```python
from build123d import *

# Parameters (mm, degrees)
SKETCH1_W                = 14.684375
SKETCH1_H                = 14.684375
BOSS_EXTRUDE1_DEPTH      = 446.0875
SKETCH9_R                = 3.384543224
CUT_EXTRUDE1_DEPTH       = 447.389511797
BOSS_EXTRUDE7_DEPTH      = 155
BOSS_EXTRUDE7_DEPTH_BACK = 155
BOSS_EXTRUDE8_DEPTH      = 164
BOSS_EXTRUDE8_DEPTH_BACK = 164
BOSS_EXTRUDE9_DEPTH      = 164
BOSS_EXTRUDE9_DEPTH_BACK = 164


with BuildPart() as part:
    # Sketch1 → Boss-Extrude1 (new body)
    with BuildSketch(Plane.XY):
        Rectangle(SKETCH1_W, SKETCH1_H)
    extrude(amount=BOSS_EXTRUDE1_DEPTH)

    # Sketch9 → Cut-Extrude1 (cut, through all)
    with BuildSketch(Plane(origin=(0, 7.3421875, 0), x_dir=(1, 0, 0), z_dir=(0, 1, 0))):
        with Locations(Location((0, -25.4, 0), (0, 0, 270))):
            Circle(SKETCH9_R)
        with Locations(Location((0, -66.675, 0), (0, 0, 270))):
            Circle(SKETCH9_R)
    extrude(amount=-CUT_EXTRUDE1_DEPTH, mode=Mode.SUBTRACT)

    # Sketch3 → Boss-Extrude7 (add, two sides: drawn at the far end of the back side and taken through both)
    with BuildSketch(Plane(origin=(0, 0, 0), x_dir=(0, 0, -1), z_dir=(1, 0, 0)).offset(-BOSS_EXTRUDE7_DEPTH_BACK)):
        with BuildLine():
            ThreePointArc((-417.5125, 0), (-422.275, 4.7625), (-427.0375, 0))
            Line((-427.0375, 0), (-417.5125, 0))
        make_face()
        with BuildLine():
            Line((-417.5125, 0), (-427.0375, 0))
            ThreePointArc((-427.0375, 0), (-422.275, -4.7625), (-417.5125, 0))
        make_face()
    extrude(amount=BOSS_EXTRUDE7_DEPTH + BOSS_EXTRUDE7_DEPTH_BACK)

    # Sketch3_3 → Boss-Extrude8 (add, two sides: drawn at the far end of the back side and taken through both)
    with BuildSketch(Plane(origin=(0, 0, 0), x_dir=(0, 0, -1), z_dir=(1, 0, 0)).offset(-BOSS_EXTRUDE8_DEPTH_BACK)):
        with BuildLine():
            ThreePointArc((-128.5875, 0), (-133.35, 4.7625), (-138.1125, 0))
            Line((-138.1125, 0), (-128.5875, 0))
        make_face()
        with BuildLine():
            Line((-128.5875, 0), (-138.1125, 0))
            ThreePointArc((-138.1125, 0), (-133.35, -4.7625), (-128.5875, 0))
        make_face()
    extrude(amount=BOSS_EXTRUDE8_DEPTH + BOSS_EXTRUDE8_DEPTH_BACK)

    # Sketch3_4 → Boss-Extrude9 (add, two sides: drawn at the far end of the back side and taken through both)
    with BuildSketch(Plane(origin=(0, 0, 0), x_dir=(0, 0, -1), z_dir=(1, 0, 0)).offset(-BOSS_EXTRUDE9_DEPTH_BACK)):
        with BuildLine():
            ThreePointArc((-290.5125, 0), (-295.275, 4.7625), (-300.0375, 0))
            Line((-300.0375, 0), (-290.5125, 0))
        make_face()
        with BuildLine():
            Line((-290.5125, 0), (-300.0375, 0))
            ThreePointArc((-300.0375, 0), (-295.275, -4.7625), (-290.5125, 0))
        make_face()
    extrude(amount=BOSS_EXTRUDE9_DEPTH + BOSS_EXTRUDE9_DEPTH_BACK)


solid = part.part
```
Check sheet for the modelled part. Datum: model origin and axes. Units: mm. A direction names the side the tool comes from. Give positions to 0.01 mm unless a question says otherwise; leave off trailing zeros. Write each loop counter-clockwise with the first axis right and the second up, starting at its lowest first coordinate (ties: lowest second). Pieces come first, ordered by that corner, then holes. Notation, with made-up numbers: (-0.5, 11.5) -> (50.5, 11.5) arc R28 cw to (50.5, 48.5) -> close; hole circle Ø3 at (73.5, 76). An arc over 180 degrees is marked (long way). Use CSV: the item, a comma, the result in double quotes. Start each with the question number.
Q1. Depth check by flat-ended pin: P1, Ø10, axis at x = 86.5, z = 288.5, coming from the +Y side; P2, Ø3, axis at y = -2, z = 100, coming from the -X side; P3, Ø5, axis at x = 44, y = 2.5, coming from the +Z side. Enter the tip coordinate at first touch or a pass-through.
Q2. Cross-section at C-C on z = 133.35. Enter the section's corners in (x, y).
Q3. Cross-section at D-D on z = 326.5. Enter the section's corners in (x, y), and give its area (3 significant figures).
Q4. Release check for a two-part mould opening along Z. For faces 5 (the flat face through (-155, 0, 422)), 6 (the flat face through (0, 0, 446.088)), 7 (the flat face through (-7.342, 0, 220)), 8 (the cylindrical face through (-82.205, -1.431, 426.818)) record: +Z half, -Z half, draft (parallel to the pull), parting line (faces both ways), or undercut.
Q5. Tool access check on faces 1 (the cylindrical face through (-86.768, -0.209, 128.592)), 2 (the cylindrical face through (84.574, 1.824, 299.674)), 3 (the flat face through (-164, 0, 295)), 4 (the flat face through (155, 0, 422)). Record the directions out of +Z, -Z, +X, -X, +Y, -Y that give a thin tool (end or side, any length) a straight path to the whole face; none if there is none.
Q6. Cross-section at A-A on y = 0. Count the separate pieces of the cut face and the enclosed holes in it, and give its area (3 significant figures).
Q7. Scan lines: line 1 along Z through (x, y) = (116.5, -4); line 2 along X through (y, z) = (0.75, 225); line 3 along Z through (x, y) = (38, -2.25). Record each from-to range of solid material in increasing order.
Working result:
1,P1,"stops at y = 4.42"
1,P2,"stops at x = -7.34"
1,P3,"stops at z = 427.04"
2,outline,"(-164, -4.76) -> (-7.34, -4.76) -> (-7.34, -7.34) -> (7.34, -7.34) -> (7.34, -4.76) -> (164, -4.76) -> (164, 4.76) -> (7.34, 4.76) -> (7.34, 7.34) -> (-7.34, 7.34) -> (-7.34, 4.76) -> (-164, 4.76) -> close"
3,outline,"(-7.34, -7.34) -> (7.34, -7.34) -> (7.34, 7.34) -> (-7.34, 7.34) -> close"
3,area,"216 mm^2"
4,face 5,"draft"
4,face 6,"+Z half"
4,face 7,"undercut"
4,face 8,"undercut"
5,face 1,"-X"
5,face 2,"+X"
5,face 3,"+Z, -Z, -X, +Y, -Y"
5,face 4,"+Z, +X, +Y, -Y"
6,separate pieces,"1"
6,enclosed holes,"2"
6,area,"15,300 mm^2"
7,line 1,"z = 130.77 to 135.93, 292.69 to 297.86, 419.69 to 424.86"
7,line 2,"x = -7.34 to 7.34"
7,line 3,"z = 129.15 to 137.55, 291.08 to 299.47, 418.08 to 426.47"
